Geometry check sheet. Reference: the model listing, model coordinates, mm. Face numbers are marked on the shaded views. A direction names the side the tool comes from. Coordinates: 2 decimals unless noted, no trailing zeros. Write each loop counter-clockwise with the first axis right and the second up, starting at its lowest first coordinate (ties: lowest second). Pieces come first, ordered by that corner, then holes.
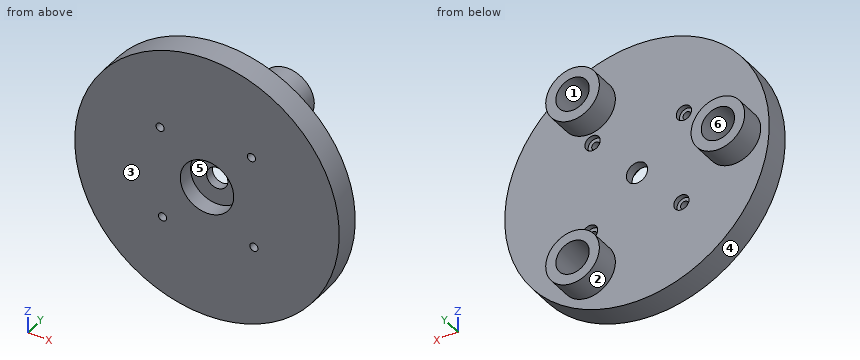
from build123d import *

# Parameters (mm, degrees)
SKETCH2_R               = 26
SKETCH2_R_2             = 2.085648148
BOSS_EXTRUDE2_DEPTH     = 10
SKETCH3_R               = 3.275
CUT_EXTRUDE1_DEPTH      = 7.5
CUT_EXTRUDE2_START      = -5
SKETCH4_R               = 26
SKETCH4_R_2             = 5.275
CUT_EXTRUDE2_DEPTH      = 5
SKETCH5_R               = 5.25
CUT_EXTRUDE3_DEPTH      = 3.2
CUT_EXTRUDE4_DEPTH      = 38.107950631
CUT_EXTRUDE4_DEPTH_BACK = 38.107950631
SKETCH6_R               = 0.8
SKETCH7_R               = 1.500000048
CUT_EXTRUDE5_DEPTH      = 1


with BuildPart() as part:
    # Sketch2 → Boss-Extrude2 (new body)
    with BuildSketch(Plane(origin=(0, 0, 0), x_dir=(1, 0, 0), z_dir=(0, 1, 0))):
        with Locations(Location((0, 0, 0), (0, 0, 270))):
            Circle(SKETCH2_R)
        with Locations(Location((0, 0, 0), (0, 0, 270))):
            Circle(SKETCH2_R_2, mode=Mode.SUBTRACT)
    extrude(amount=BOSS_EXTRUDE2_DEPTH)

    # Sketch3 → Cut-Extrude1 (cut)
    with BuildSketch(Plane.XZ.offset(-10)):
        with Locations(Location((9.52625, -16.499949006, 0), (0, 0, 270))):
            Circle(SKETCH3_R)
        with Locations(Location((9.52625, 16.499949006, 0), (0, 0, 270))):
            Circle(SKETCH3_R)
        with Locations(Location((-19.0525, 0, 0), (0, 0, 270))):
            Circle(SKETCH3_R)
    extrude(amount=CUT_EXTRUDE1_DEPTH, mode=Mode.SUBTRACT)

    # Sketch4 → Cut-Extrude2 (cut)
    with BuildSketch(Plane(origin=(0, 10, 0), x_dir=(1, 0, 0), z_dir=(0, 1, 0)).offset(CUT_EXTRUDE2_START)):
        with Locations(Location((0, 0, 0), (0, 0, 270))):
            Circle(SKETCH4_R)
        with Locations(Location((-19.0525, 0, 0), (0, 0, 270))):
            Circle(SKETCH4_R_2, mode=Mode.SUBTRACT)
        with Locations(Location((9.52625, -16.499949006, 0), (0, 0, 270))):
            Circle(SKETCH4_R_2, mode=Mode.SUBTRACT)
        with Locations(Location((9.52625, 16.499949006, 0), (0, 0, 270))):
            Circle(SKETCH4_R_2, mode=Mode.SUBTRACT)
    extrude(amount=CUT_EXTRUDE2_DEPTH, mode=Mode.SUBTRACT)

    # Sketch5 → Cut-Extrude3 (cut)
    with BuildSketch(Plane.XZ):
        with Locations(Location((0, 0, 0), (0, 0, 270))):
            Circle(SKETCH5_R)
    extrude(amount=-CUT_EXTRUDE3_DEPTH, mode=Mode.SUBTRACT)

    # Sketch6 → Cut-Extrude4 (cut, two sides: drawn at the far end of the back side and taken through both)
    with BuildSketch(Plane(origin=(0, 5, 0), x_dir=(1, 0, 0), z_dir=(0, 1, 0)).offset(-CUT_EXTRUDE4_DEPTH_BACK)):
        with Locations(Location((-8.733127343, 9.220763895, 0), (0, 0, 270))):
            Circle(SKETCH6_R)
        with Locations(Location((9.220763895, 8.733127343, 0), (0, 0, 270))):
            Circle(SKETCH6_R)
        with Locations(Location((8.733127343, -9.220763895, 0), (0, 0, 270))):
            Circle(SKETCH6_R)
        with Locations(Location((-9.220763895, -8.733127343, 0), (0, 0, 270))):
            Circle(SKETCH6_R)
    extrude(amount=CUT_EXTRUDE4_DEPTH + CUT_EXTRUDE4_DEPTH_BACK, mode=Mode.SUBTRACT)

    # Sketch7 → Cut-Extrude5 (cut)
    with BuildSketch(Plane(origin=(0, 5, 0), x_dir=(1, 0, 0), z_dir=(0, 1, 0))):
        with Locations(Location((-8.733127343, 9.220763895, 0), (0, 0, 270))):
            Circle(SKETCH7_R)
        with Locations(Location((9.220763895, 8.733127343, 0), (0, 0, 270))):
            Circle(SKETCH7_R)
        with Locations(Location((8.733127343, -9.220763895, 0), (0, 0, 270))):
            Circle(SKETCH7_R)
        with Locations(Location((-9.220763895, -8.733127343, 0), (0, 0, 270))):
            Circle(SKETCH7_R)
    extrude(amount=-CUT_EXTRUDE5_DEPTH, mode=Mode.SUBTRACT)


solid = part.part
1. Sectioned sample at D-D, the plane x = 16. Record the boundary of the cut face in (y, z), and give its area (3 significant figures).
Computed values:
outline: (0, -20.49) - (5, -20.49) - (5, 20.49) - (0, 20.49) - close
area: 205 mm2
2. Access from +Z, -Z, +X, -X, +Y, -Y to the whole of each face (thin tool, end or side, straight path). Record for the marked faces 5 and 6.
Computed values:
face 5: -Y
face 6: +Y
3. Sectioned sample at C-C, the plane z = 15.5. Record the boundary of the cut face in (x, y), and give its area (3 significant figures).
Computed values:
outline: (-20.87, 0) - (20.87, 0) - (20.87, 5) - (14.71, 5) - (14.71, 10) - (12.64, 10) - (12.64, 2.5) - (6.41, 2.5) - (6.41, 10) - (4.35, 10) - (4.35, 5) - (-20.87, 5) - close
area: 214 mm2
4. Gauge pin test, flat ends, axial feed: pin 1 Ø6 at (x, y) = (12.5, 1) entering from -Z; pin 2 Ø5 at (x, y) = (-0.5, 8.5) entering from +Z; pin 3 Ø2 at (y, z) = (3, -2) entering from -X; pin 4 Ø3 at (y, z) = (5, -1) entering from +X. Record the tip position at first contact, or that the pin passes through.
Computed values:
pin 1: stops at z = -24.2
pin 2: passes through
pin 3: stops at x = -25.98
pin 4: stops at x = 26
5. Sectioned sample at A-A, the plane x = 0. Record the boundary of the cut face in (y, z), and give its area (3 significant figures).
Computed values:
outline: (0, -26) - (5, -26) - (5, -2.09) - (3.2, -2.09) - (3.2, -5.25) - (0, -5.25) - close; (0, 5.25) - (3.2, 5.25) - (3.2, 2.09) - (5, 2.09) - (5, 26) - (0, 26) - close
area: 219 mm2
6. Thickness scan on line 1 along X through (y, z) = (2.75, 0); line 2 along X through (y, z) = (8.75, 0); line 3 along Y through (x, z) = (11.5, 8). Record the ranges inside material, lowest first.
Computed values:
line 1: x = -26 to -22.33, -15.78 to -5.25, 5.25 to 26
line 2: x = -24.33 to -22.33, -15.78 to -13.78
line 3: y = 0 to 5
7. Sectioned sample at B-B, the plane z = 0. Record the boundary of the cut face in (x, y).
Computed values:
outline: (-26, 0) - (-5.25, 0) - (-5.25, 3.2) - (-2.09, 3.2) - (-2.09, 5) - (-13.78, 5) - (-13.78, 10) - (-15.78, 10) - (-15.78, 2.5) - (-22.33, 2.5) - (-22.33, 10) - (-24.33, 10) - (-24.33, 5) - (-26, 5) - close; (2.09, 3.2) - (5.25, 3.2) - (5.25, 0) - (26, 0) - (26, 5) - (2.09, 5) - close
8. Draft check along Z on the marked faces 1, 2, 3 and 4. Enter one of: released by +Z, released by -Z, zero draft, split by the parting line, or undercut.
Computed values:
face 1: undercut
face 2: undercut
face 3: zero draft
face 4: split by the parting line
